```python
from build123d import *

# Parameters (mm, degrees)
SZKIC1_W                    = 5
SZKIC1_H                    = 6
SZKIC1_W_2                  = 2.1
SZKIC1_H_2                  = 2.1
DODANIE_WYCI_GNI_CIE1_DEPTH = 4
SZKIC3_W                    = 6.5
SZKIC3_H                    = 14
DODANIE_WYCI_GNI_CIE2_DEPTH = 3
WYTNIJ_WYCI_GNI_CIE1_DEPTH  = 13.492097502


with BuildPart() as part:
    # Szkic1 → Dodanie-wyciągnięcie1 (new body)
    with BuildSketch(Plane.XY):
        with Locations((1.05, -1.05)):
            Rectangle(SZKIC1_W, SZKIC1_H)
        with Locations((1.05, -1.05)):
            Rectangle(SZKIC1_W_2, SZKIC1_H_2, mode=Mode.SUBTRACT)
    extrude(amount=DODANIE_WYCI_GNI_CIE1_DEPTH)

    # Szkic3 → Dodanie-wyciągnięcie2 (add)
    with BuildSketch(Plane.XY.offset(4)):
        with Locations((1.05, -1.05)):
            Rectangle(SZKIC3_W, SZKIC3_H)
    extrude(amount=DODANIE_WYCI_GNI_CIE2_DEPTH)

    # Szkic4 → Wytnij-wyciągnięcie1 (cut, through all)
    with BuildSketch(Plane.ZY.offset(2.2)):
        with BuildLine():
            Line((7, -8.05), (7, -1.05))
            add(Edge.make_bspline(
                [(7, -1.05), (7, -4.55), (5.5, -8.05)],
                knots=[0.5, 0.5, 0.5, 1, 1, 1], degree=2))
            Line((5.5, -8.05), (7, -8.05))
        make_face()
        with BuildLine():
            Line((7, 5.95), (5.5, 5.95))
            add(Edge.make_bspline(
                [(5.5, 5.95), (7, 2.45), (7, -1.05)],
                knots=[0, 0, 0, 0.5, 0.5, 0.5], degree=2))
            Line((7, -1.05), (7, 5.95))
        make_face()
    extrude(amount=-WYTNIJ_WYCI_GNI_CIE1_DEPTH, mode=Mode.SUBTRACT)


solid = part.part
```
Source: CAD feature listing. Evaluate the final solid. Frame: model axes, mm. A direction names the side the tool comes from. Round coordinates to 2 decimals unless told otherwise and drop trailing zeros. Loops run counter-clockwise (first coordinate to the right, second up) from the corner with the lowest first, then second, coordinate; pieces in that order, holes last. Notation, with made-up numbers: M 27.5,29.5 L 75.5,29.5 A26 cw 75.5,54.5 Z; hole C 82.25,-23 d8. An arc over 180 degrees is marked long. Use a Markdown table: item, result. Add a question column.
1. Pull-direction query (X, two-part tool) for faces 5 (the flat face through (3.55, -1, 2)), 6 (the flat face through (1, -2.1, 2)), 7 (the flat face through (1, 5.95, 5)); classes: +X half, -X half, draft (parallel to the pull), parting line (faces both ways), or undercut.
2. Ray query, line 1 along Y through (x, z) = (0.5, 2.5); line 2 along Z through (x, y) = (1.25, -0.75); line 3 along X through (y, z) = (1.75, 1.75). Return the intervals inside material, ascending. Write a range as [from, to].
3. Contact query for flat-ended pins moving along their axis: pin 1 (1.7 mm diameter, centred on y = -1, z = 2, fed in from +X); pin 2 (0.6 mm diameter, centred on x = 1.5, z = 2.5, fed in from -Y); pin 3 (1.7 mm diameter, centred on y = -1, z = 3, fed in from -X); pin 4 (2 mm diameter, centred on y = -6.5, z = 2.5, fed in from -X). Output: stop coordinate, or through.
4. Cut plane A-A, the plane z = 2. Output: boundary loops of the cut face in (x, y).
5. Set-up query: faces 1 (the flat face through (1, 1.95, 2)), 2 (the flat face through (1, -1, 4)), 3 (the flat face through (1, -4.05, 2)), 4 (the flat face through (-1.45, -1, 2)). Return all of +Z, -Z, +X, -X, +Y, -Y with unobstructed straight access to the full face (end or side cutting, diameter ignored); none if empty.
Solution:
| question | item | result |
|---|---|---|
| 1 | face 5 | +X half |
| 1 | face 6 | undercut |
| 1 | face 7 | draft |
| 2 | line 1 | y = [-4.05, -2.1], [0, 1.95] |
| 2 | line 2 | z = [4, 7] |
| 2 | line 3 | x = [-1.45, 3.55] |
| 3 | pin 1 | stops at x = 3.55 |
| 3 | pin 2 | stops at y = -4.05 |
| 3 | pin 3 | stops at x = -1.45 |
| 3 | pin 4 | passes through |
| 4 | outline | M -1.45,-4.05 L 3.55,-4.05 L 3.55,1.95 L -1.45,1.95 Z; hole M 0,-2.1 L 2.1,-2.1 L 2.1,0 L 0,0 Z |
| 5 | face 1 | -Z, +X, -X, +Y |
| 5 | face 2 | -Z |
| 5 | face 3 | -Z, +X, -X, -Y |
| 5 | face 4 | -Z, -X, +Y, -Y |
